from build123d import *

# Parameters (mm, degrees)
BOSS_EXTRU_1_DEPTH = 5
CONG_1_R           = 0.5


with BuildPart() as part:
    # Esquisse1 → Boss.-Extru.1 (new, symmetric)
    with BuildSketch(Plane.XY):
        Polygon((-15, 8), (0, 8), (0, 0), (-19.618802154, 0), align=None)
    extrude(amount=BOSS_EXTRU_1_DEPTH, both=True)

    # Congé1
    cong_1_edges = [part.edges().sort_by_distance(p)[0] for p in [
        (-15, 8, 0),
        (0, 8, 0),
    ]]
    fillet(cong_1_edges, radius=CONG_1_R)


solid = part.part
Could you check a few things on this model? Use its own coordinates, in mm. Coordinates: 2 decimals unless noted, no trailing zeros. Order: outer loops, then holes, each group sorted by start corner. A loop starts at its lowest first (then second) coordinate and runs counter-clockwise, first axis right, second up.
Q1. Suppose I cut it at B-B on y = 6.75. Please give me the cut outline in (x, z), and give its area (3 significant figures).
Q2. Please list where these lines run through material, in increasing order: L1, parallel to X at y = 5.75, z = -3; L2, parallel to X at y = 7.25, z = 0.5.
Q3. Suppose I cut it at A-A on z = 4.5. Please give me the cut outline in (x, y).
Q4. Suppose I cut it at C-C on y = 3.75. Please give me the cut outline in (x, z), and give its area (3 significant figures).
Answer:
1. outline: (-15.72, -5) - (0, -5) - (0, 5) - (-15.72, 5) - close
1. area: 157 mm2
2. L1: x = -16.3 to 0
2. L2: x = -15.43 to 0
3. outline: (-19.62, 0) - (0, 0) - (0, 7.5) arc R0.5 ccw to (-0.5, 8) - (-14.71, 8) arc R0.5 ccw to (-15.14, 7.75) - close
4. outline: (-17.45, -5) - (0, -5) - (0, 5) - (-17.45, 5) - close
4. area: 175 mm2
